```python
from build123d import *

# Parameters (mm, degrees)
SCHIZZO2_R                   = 10.5
ESTRUSIONE_ESTRUSIONE1_DEPTH = 8
TAGLIO_ESTRUSIONE1_START     = -2
TAGLIO_ESTRUSIONE1_DEPTH     = 2
TAGLIO_ESTRUSIONE2_START     = -3.1
SCHIZZO4_R                   = 4.75
TAGLIO_ESTRUSIONE2_DEPTH     = 3.1
TAGLIO_ESTRUSIONE4_START     = -1.9
SCHIZZO5_R                   = 9
SCHIZZO5_R_2                 = 4.75
TAGLIO_ESTRUSIONE4_DEPTH     = 1.9
SCHIZZO6_R                   = 3
ESTRUSIONE_ESTRUSIONE2_DEPTH = 3
TAGLIO_ESTRUSIONE5_DEPTH     = 2.48
FORO_PER_VITE_M2_1_D         = 2.6


with BuildPart() as part:
    # Schizzo2 → Estrusione-Estrusione1 (new body)
    with BuildSketch(Plane(origin=(0, 0, 0), x_dir=(1, 0, 0), z_dir=(0, 1, 0))):
        with Locations(Location((0, 0, 0), (0, 0, 270))):
            Circle(SCHIZZO2_R)
    extrude(amount=ESTRUSIONE_ESTRUSIONE1_DEPTH)

    # Schizzo3 → Taglio-Estrusione1 (cut)
    with BuildSketch(Plane(origin=(0, 8, 0), x_dir=(1, 0, 0), z_dir=(0, 1, 0)).offset(TAGLIO_ESTRUSIONE1_START)):
        with BuildLine():
            Line((8.146740146, 3.825), (9.50453017, 4.4625))
            ThreePointArc((9.50453017, 4.4625), (-10.5, 0), (9.50453017, -4.4625))
            Line((9.50453017, -4.4625), (8.146740146, -3.825))
            ThreePointArc((8.146740146, -3.825), (9, 0), (8.146740146, 3.825))
        make_face()
    extrude(amount=TAGLIO_ESTRUSIONE1_DEPTH, mode=Mode.SUBTRACT)

    # Schizzo4 → Taglio-Estrusione2 (cut)
    with BuildSketch(Plane(origin=(0, 6, 0), x_dir=(1, 0, 0), z_dir=(0, 1, 0)).offset(TAGLIO_ESTRUSIONE2_START)):
        with BuildLine():
            Line((8.146740146, 3.825), (9.50453017, 4.4625))
            ThreePointArc((9.50453017, 4.4625), (-10.5, 0), (9.50453017, -4.4625))
            Line((9.50453017, -4.4625), (8.146740146, -3.825))
            ThreePointArc((8.146740146, -3.825), (9, 0), (8.146740146, 3.825))
        make_face()
        with Locations(Location((0, 0, 0), (0, 0, 270))):
            Circle(SCHIZZO4_R, mode=Mode.SUBTRACT)
    extrude(amount=TAGLIO_ESTRUSIONE2_DEPTH, mode=Mode.SUBTRACT)

    # Schizzo5 → Taglio-Estrusione4 (cut)
    with BuildSketch(Plane(origin=(0, 2.9, 0), x_dir=(1, 0, 0), z_dir=(0, 1, 0)).offset(TAGLIO_ESTRUSIONE4_START)):
        with Locations(Location((0, 0, 0), (0, 0, 270))):
            Circle(SCHIZZO5_R)
        with Locations(Location((0, 0, 0), (0, 0, 270))):
            Circle(SCHIZZO5_R_2, mode=Mode.SUBTRACT)
    extrude(amount=TAGLIO_ESTRUSIONE4_DEPTH, mode=Mode.SUBTRACT)

    # Schizzo6 → Estrusione-Estrusione2 (add)
    with BuildSketch(Plane(origin=(0, 6, 0), x_dir=(1, 0, 0), z_dir=(0, 1, 0))):
        with Locations(Location((0, 0, 0), (0, 0, 270))):
            Circle(SCHIZZO6_R)
    extrude(amount=ESTRUSIONE_ESTRUSIONE2_DEPTH)

    # Schizzo7 → Taglio-Estrusione5 (cut)
    with BuildSketch(Plane.XZ):
        with BuildLine():
            Line((1.5, -2.598076211), (1.5, 2.598076211))
            ThreePointArc((1.5, 2.598076211), (-3, 0), (1.5, -2.598076211))
        make_face()
    extrude(amount=-TAGLIO_ESTRUSIONE5_DEPTH, mode=Mode.SUBTRACT)

    # Foro per Vite M2-1 (through all)
    with Locations(Plane(origin=(0, 9, 0), x_dir=(1, 0, 0), z_dir=(0, 1, 0))):
        with Locations((0, 0)):
            Hole(FORO_PER_VITE_M2_1_D / 2)


solid = part.part
```
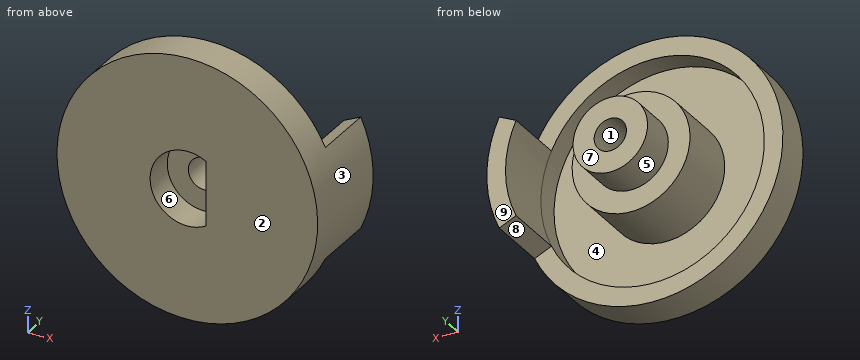
For this review, take the finished solid that the model builds, in its own axes (mm). Face numbers are marked on the shaded views. A direction names the side the tool comes from. Round coordinates to 2 decimals unless told otherwise and drop trailing zeros. Write each loop counter-clockwise with the first axis right and the second up, starting at its lowest first coordinate (ties: lowest second). Pieces come first, ordered by that corner, then holes. Notation, with made-up numbers: (25.25, -23.5) -> (60.25, -23.5) arc R22 ccw to (60.25, -6.5) -> close; hole circle Ø4 at (89.25, -2). An arc over 180 degrees is marked (long way). One line per question, with ' | ' between items. Start each with the question number.
(1) Add section C-C, the plane y = 7.75. Write out the cut boundary in (x, z) (1 decimal).
(2) Add section A-A, the plane y = 1.5. Write out the cut boundary in (x, z), plus the area to 3 significant figures.
(3) Add section B-B, the plane z = 0. Write out the cut boundary in (x, y), plus the area to 3 significant figures.
(4) Tool access review of the marked faces 5, 6, 7, 8 and 9: name each direction out of +Z, -Z, +X, -X, +Y, -Y from which nothing blocks a thin tool from reaching the whole face with its end or side.
(5) Mouldability with a two-part tool opening along Z and no side actions: class the marked faces 1, 2, 3 and 4 as released by +Z, released by -Z, zero draft, split by the parting line, or undercut.
(6) Add section D-D, the plane x = 0. Write out the cut boundary in (y, z), plus the area to 3 significant figures.
(7) For line 1 along X through (y, z) = (2.3, 0); line 2 along X through (y, z) = (2, 3.5); line 3 along X through (y, z) = (0.7, 0), list the stretches that pass through material, from the lowest coordinate up. Write a range as from..to.
(8) Insertion check: P1, Ø1, axis at y = 1, z = 4.5, coming from the +X side; P2, Ø1.9, axis at x = 9.5, z = 0.5, coming from the +Y side; P3, Ø10, axis at x = -7.5, z = 6.5, coming from the +Y side. Each pin has a flat end and moves straight along its axis. Give the tip position at first contact, or say it passes through.
Answer list:
1) outline: circle Ø6 at (0, 0); (8.1, -3.8) -> (9.5, -4.5) arc R10.5 ccw to (9.5, 4.5) -> (8.1, 3.8) arc R9 cw to start; hole circle Ø2.6 at (0, 0)
2) outline: circle Ø21 at (0, 0); circle Ø9.5 at (0, 0); hole circle Ø18 at (0, 0); hole (1.5, -2.6) -> (1.5, 2.6) arc R3 ccw (long way) to start | area: 140 mm²
3) outline: (-10.5, 0) -> (-3, 0) -> (-3, 2.48) -> (-1.3, 2.48) -> (-1.3, 9) -> (-3, 9) -> (-3, 6) -> (-4.75, 6) -> (-4.75, 1) -> (-9, 1) -> (-9, 2.9) -> (-10.5, 2.9) -> close; (1.3, 2.48) -> (1.5, 2.48) -> (1.5, 0) -> (10.5, 0) -> (10.5, 8) -> (9, 8) -> (9, 1) -> (4.75, 1) -> (4.75, 6) -> (3, 6) -> (3, 9) -> (1.3, 9) -> close | area: 71.7 mm²
4) face 5: +Y | face 6: -Y | face 7: +Z, -Z, +X, -X, +Y | face 8: -Z, +Y | face 9: +Z, -Z, +X, +Y
5) face 1: undercut | face 2: zero draft | face 3: split by the parting line | face 4: undercut
6) outline: (0, -10.5) -> (2.9, -10.5) -> (2.9, -9) -> (1, -9) -> (1, -4.75) -> (6, -4.75) -> (6, -3) -> (9, -3) -> (9, -1.3) -> (2.48, -1.3) -> (2.48, -3) -> (0, -3) -> close; (0, 3) -> (2.48, 3) -> (2.48, 1.3) -> (9, 1.3) -> (9, 3) -> (6, 3) -> (6, 4.75) -> (1, 4.75) -> (1, 9) -> (2.9, 9) -> (2.9, 10.5) -> (0, 10.5) -> close | area: 60.4 mm²
7) line 1: -10.5..-9, -4.75..-3, 1.5..4.75, 9..10.5 | line 2: -9.9..-8.29, -3.21..3.21, 8.29..9.9 | line 3: -10.5..-3, 1.5..10.5
8) P1: x = 9.71 | P2: y = 8 | P3: y = 2.9
